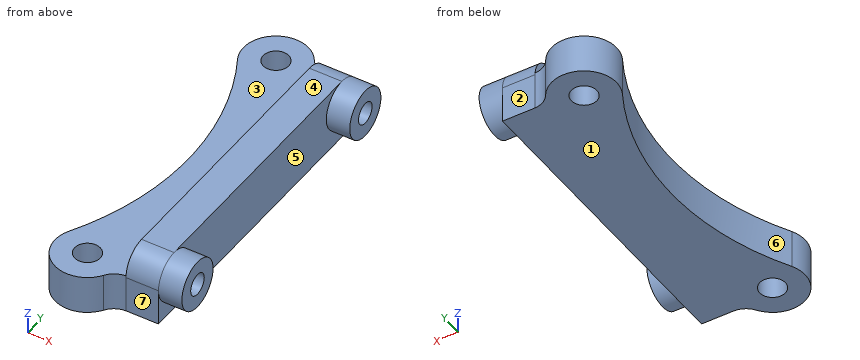
from build123d import *

# Parameters (mm, degrees)
EXTRUDE1_DEPTH     = 15.875
SKETCH2_R          = 12.065
EXTRUDE2_DEPTH     = 11.43
EXTRUDE4_DEPTH     = 18.796
SKETCH5_R          = 6.2484
CUT_EXTRUDE1_DEPTH = 19.796
SKETCH7_R          = 5.25018
CUT_EXTRUDE2_DEPTH = 25.4


with BuildPart() as part:
    # Sketch1 → Extrude1 (new body)
    with BuildSketch(Plane(origin=(0, 0, 0), x_dir=(0, 0, -1), z_dir=(1, 0, 0))):
        with BuildLine():
            Line((17.907, -77.0636), (17.907, 77.0636))
            Line((17.907, 77.0636), (0, 77.0636))
            ThreePointArc((0, 77.0636), (-8.531243315, 73.529843315), (-12.065, 64.9986))
            Line((-12.065, 64.9986), (-12.065, -64.9986))
            ThreePointArc((-12.065, -64.9986), (-8.531243315, -73.529843315), (0, -77.0636))
            Line((0, -77.0636), (17.907, -77.0636))
        make_face()
    extrude(amount=EXTRUDE1_DEPTH)

    # Sketch2 → Extrude2 (add)
    with BuildSketch(Plane(origin=(15.875, 0, 0), x_dir=(0, 0, -1), z_dir=(1, 0, 0))):
        with Locations(Location((0, 64.9986, 0), (0, 0, 180))):  # turned: the seam where the file's is
            Circle(SKETCH2_R)
    extrude2 = extrude(amount=EXTRUDE2_DEPTH)

    # Mirror of Extrude 2: Extrude2 across plane
    add(extrude2.mirror(Plane.ZX))

    # Sketch4 → Extrude4 (add)
    with BuildSketch(Plane(origin=(0, 0, -17.907), x_dir=(-1, 0, 0), z_dir=(0, 0, -1))):
        with BuildLine():
            ThreePointArc((8.015455062, 81.59619111), (4.56701856, 78.340842715), (0, 77.0636))
            Line((0, 77.0636), (0, -77.0636))
            ThreePointArc((0, -77.0636), (4.56701856, -78.340842715), (8.015455062, -81.59619111))
            ThreePointArc((8.015455062, -81.59619111), (29.290525196, -86.75258508), (35.488071258, -65.757170562))
            ThreePointArc((35.488071258, -65.757170562), (18.264230861, 0), (35.488071258, 65.757170562))
            ThreePointArc((35.488071258, 65.757170562), (29.290525196, 86.75258508), (8.015455062, 81.59619111))
        make_face()
    extrude(amount=-EXTRUDE4_DEPTH)

    # Sketch5 → Cut-Extrude1 (cut, through all)
    with BuildSketch(Plane.XY.offset(0.889)):
        with Locations((-21.3614, 72.9996)):
            Circle(SKETCH5_R)
    cut_extrude1 = extrude(amount=-CUT_EXTRUDE1_DEPTH, mode=Mode.SUBTRACT)

    # Sketch7 → Cut-Extrude2 (cut)
    with BuildSketch(Plane(origin=(27.305, 0, 0), x_dir=(0, 0, -1), z_dir=(1, 0, 0))):
        with Locations((0, 64.9986)):
            Circle(SKETCH7_R)
    cut_extrude2 = extrude(amount=-CUT_EXTRUDE2_DEPTH, mode=Mode.SUBTRACT)

    # Mirror1: Cut-Extrude1, Cut-Extrude2 across plane
    add(cut_extrude1.mirror(Plane.ZX), mode=Mode.SUBTRACT)
    add(cut_extrude2.mirror(Plane.ZX), mode=Mode.SUBTRACT)


solid = part.part
Model file for the job. Use its own axes, mm. Face numbers are marked on the shaded views. A direction names the side the tool comes from. Give positions to 0.01 mm unless a question says otherwise; leave off trailing zeros. Loops run counter-clockwise (first coordinate to the right, second up) from the corner with the lowest first, then second, coordinate; pieces in that order, holes last.
Item 1: Drop flat-ended pins along their axis: P1, Ø13.5, axis at y = 65, z = 0, coming from the -X side; P2, Ø12, axis at x = 14.5, z = 7.5, coming from the +Y side; P3, Ø10, axis at x = -10, y = 15.5, coming from the +Z side; P4, Ø11, axis at x = -21.36, y = -73, coming from the -Z side. Give the stop position or say it passes through.
Check values:
P1: stops at x = -37.19
P2: stops at y = 76.97
P3: stops at z = 0.89
P4: passes through
Item 2: Mould opens along Y. For the marked faces 4, 5, 6 and 7 say: +Y half, -Y half, draft (parallel to the pull), parting line (faces both ways), or undercut.
Check values:
face 4: draft
face 5: undercut
face 6: undercut
face 7: -Y half
Item 3: Drill centre lines: line 1 along Y through (x, z) = (16.5, 0); line 2 along Y through (x, z) = (16.5, -4); line 3 along Y through (x, z) = (-17, -11). Where is each one in solid material? Low to high.
Check values:
line 1: y = -77.06 to -70.25, -59.75 to -52.93, 52.93 to 59.75, 70.25 to 77.06
line 2: y = -76.38 to -68.4, -61.6 to -53.62, 53.62 to 61.6, 68.4 to 76.38
line 3: y = -88.26 to -77.47, -68.53 to 68.53, 77.47 to 88.26
Item 4: Slice it at D-D (y = -12.5). Write the cut outline in (x, z) (3 decimals).
Check values:
outline: (-18.848, -17.907) - (15.875, -17.907) - (15.875, 12.065) - (0, 12.065) - (0, 0.889) - (-18.848, 0.889) - close
Item 5: Slice it at B-B (x = 5.5). Write the cut outline in (y, z) (3 decimals).
Check values:
outline: (-77.064, -17.907) - (77.064, -17.907) - (77.064, 0) arc R12.065 ccw to (64.999, 12.065) - (-64.999, 12.065) arc R12.065 ccw to (-77.064, 0) - close; hole circle Ø10.5 at (-64.999, 0); hole circle Ø10.5 at (64.999, 0)
Item 6: Slice it at C-C (z = -8.75). Write the cut outline in (x, y) (3 decimals), plus the area to 3 significant figures.
Check values:
outline: (-35.488, -65.757) arc R15.875 ccw to (-8.015, -81.596) arc R9.896 cw to (0, -77.064) - (15.875, -77.064) - (15.875, -73.305) - (27.305, -73.305) - (27.305, -56.692) - (15.875, -56.692) - (15.875, 56.692) - (27.305, 56.692) - (27.305, 73.305) - (15.875, 73.305) - (15.875, 77.064) - (0, 77.064) arc R9.896 cw to (-8.015, 81.596) arc R15.875 ccw to (-35.488, 65.757) arc R134.136 cw to start; hole circle Ø12.497 at (-21.361, -73); hole circle Ø12.497 at (-21.361, 73)
area: 7,100 mm2
Item 7: Which spindle directions (+Z, -Z, +X, -X, +Y, -Y) get a long thin tool onto all of the face, cutting with end or side? Do the marked faces 1, 2 and 3. Say none if no direction does.
Check values:
face 1: -Z, +X, -X, +Y, -Y
face 2: +Z, -Z, +X, +Y
face 3: +Z, -X, +Y, -Y
Item 8: Slice it at A-A (x = 22.5). Write the cut outline in (y, z) (3 decimals).
Check values:
outline: circle Ø24.13 at (-64.999, 0); circle Ø24.13 at (64.999, 0); hole circle Ø10.5 at (-64.999, 0); hole circle Ø10.5 at (64.999, 0)
